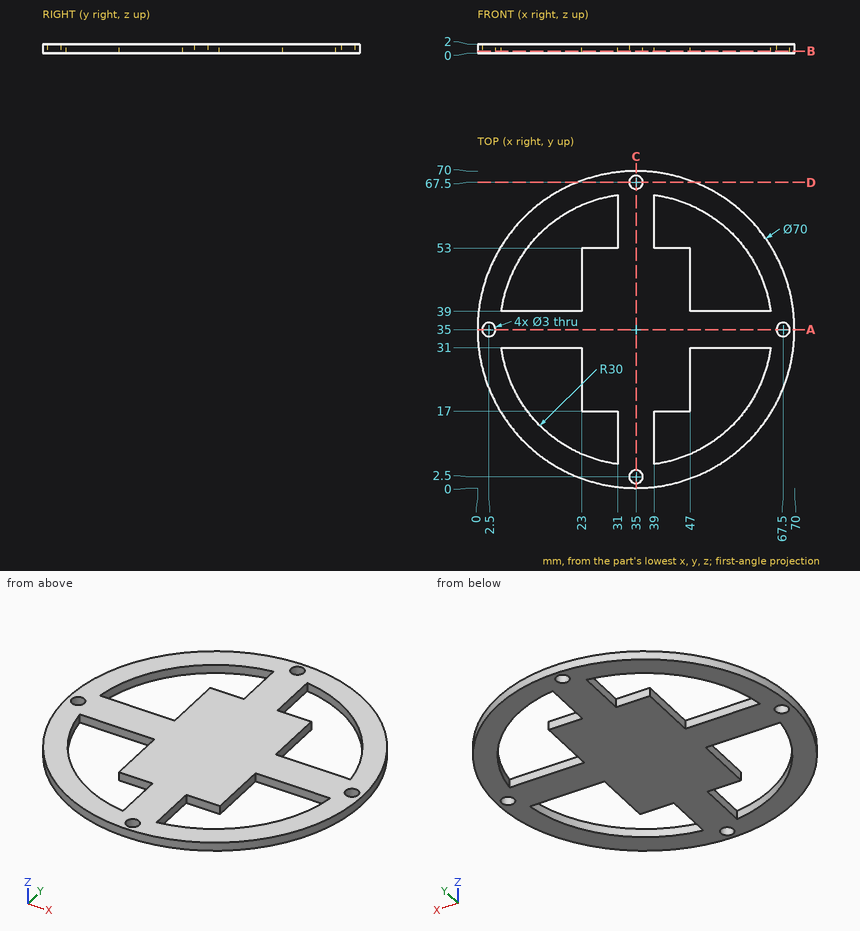
Geometry: see drawing. Coordinates: mm, zero at the bounding-box minimum. Give positions to 0.01 mm unless a question says otherwise; leave off trailing zeros. Loops run counter-clockwise (first coordinate to the right, second up) from the corner with the lowest first, then second, coordinate; pieces in that order, holes last. Notation, with made-up numbers: (35, -24) - (80, -24) arc R28 cw to (80, 0) - close; hole circle Ø10 at (86.5, -30). An arc over 180 degrees is marked (long way). Use CSV: the item, a comma, the result in double quotes. Start each with the question number.
Item 1: Section A-A on y = 35. Return loops of the section in (x, z), then the cut area to 3 significant figures.
Item 2: Contact query for flat-ended pins moving along their axis: P1, Ø1, axis at y = 56.5, z = 1, coming from the -X side; P2, Ø1, axis at x = 48.5, z = 1, coming from the +Y side; P3, Ø0.6, axis at y = 13, z = 1, coming from the +X side. Output: stop coordinate, or through.
Item 3: Line query: line 1 (Y direction, x = 35, z = 0.7); line 2 (X direction, y = 58.5, z = 0.75); line 3 (Y direction, x = 45, z = 0.8). Output: solid intervals per line, ascending.
Item 4: Section B-B on z = 0.4. State how many separate pieces and enclosed holes the cut face has, then the cut area to 3 significant figures.
Item 5: Section D-D on y = 67.5. Return loops of the section in (x, z), then the cut area to 3 significant figures.
Ans:
1,outline,"(0, 0) - (1, 0) - (1, 2) - (0, 2) - close; (4, 0) - (66, 0) - (66, 2) - (4, 2) - close; (69, 0) - (70, 0) - (70, 2) - (69, 2) - close"
1,area,"128 mm2"
2,P1,"stops at x = 7"
2,P2,"stops at y = 67.5"
2,P3,"stops at x = 62.46"
3,line 1,"y = 0 to 1, 4 to 66, 69 to 70"
3,line 2,"x = 9.06 to 16.35, 31 to 39, 53.65 to 60.94"
3,line 3,"y = 1.46 to 6.72, 17 to 53, 63.28 to 68.54"
4,separate pieces,"1"
4,enclosed holes,"8"
4,area,"2,330 mm2"
5,outline,"(22.01, 0) - (33.5, 0) - (33.5, 2) - (22.01, 2) - close; (36.5, 0) - (47.99, 0) - (47.99, 2) - (36.5, 2) - close"
5,area,"46.0 mm2"
